```python
from build123d import *

# Parameters (mm, degrees)
SKETCH1_R           = 105
SKETCH1_R_2         = 20.325
BOSS_EXTRUDE1_DEPTH = 10
SKETCH2_R           = 6
CUT_EXTRUDE1_DEPTH  = 10
CIRPATTERN1_COUNT   = 6
SKETCH4_R           = 6
CUT_EXTRUDE2_DEPTH  = 10


with BuildPart() as part:
    # Sketch1 → Boss-Extrude1 (new body)
    with BuildSketch(Plane(origin=(0, 0, 0), x_dir=(1, 0, 0), z_dir=(0, 1, 0))):
        with Locations(Location((0, 0, 0), (0, 0, 270))):
            Circle(SKETCH1_R)
        with Locations(Location((0, 0, 0), (0, 0, 270))):
            Circle(SKETCH1_R_2, mode=Mode.SUBTRACT)
    extrude(amount=BOSS_EXTRUDE1_DEPTH)

    # Sketch2 → Cut-Extrude1 (cut)
    with BuildSketch(Plane(origin=(0, 10, 0), x_dir=(1, 0, 0), z_dir=(0, 1, 0))):
        with Locations(Location((93.00155101, 0.192929613, 0), (0, 0, 270))):
            Circle(SKETCH2_R)
        with Locations(Location((-46.333693559, -80.638170573, 0), (0, 0, 270))):
            Circle(SKETCH2_R)
        with Locations(Location((-46.667857451, 80.445240959, 0), (0, 0, 270))):
            Circle(SKETCH2_R)
    cut_extrude1 = extrude(amount=-CUT_EXTRUDE1_DEPTH, mode=Mode.SUBTRACT)

    # CirPattern1: Cut-Extrude1 ×6 about axis
    cirpattern1_axis = Axis((0, 0, 0), (0, 1, 0))
    for i in range(1, CIRPATTERN1_COUNT):
        add(cut_extrude1.rotate(cirpattern1_axis, i * 360 / CIRPATTERN1_COUNT), mode=Mode.SUBTRACT)

    # Sketch4 → Cut-Extrude2 (cut)
    with BuildSketch(Plane(origin=(0, 10, 0), x_dir=(1, 0, 0), z_dir=(0, 1, 0))):
        with Locations(Location((0, 80, 0), (0, 0, 270))):
            Circle(SKETCH4_R)
    extrude(amount=-CUT_EXTRUDE2_DEPTH, mode=Mode.SUBTRACT)


solid = part.part
```
The model under review builds one solid part; all positions refer to its coordinate system, in mm. Round coordinates to 2 decimals unless told otherwise and drop trailing zeros. Loops run counter-clockwise (first coordinate to the right, second up) from the corner with the lowest first, then second, coordinate; pieces in that order, holes last. Notation, with made-up numbers: (54, -14.75) -> (104, -14.75) arc R17 cw to (104, 14.25) -> close; hole circle Ø7 at (-5.75, 39.5). An arc over 180 degrees is marked (long way). Answer in a Markdown table with one row per item.
1) Consider section D-D, the plane y = 6.75. Count the separate pieces of the cut face and the enclosed holes in it, plus the area to 3 significant figures.
Taken from the geometry:
| item | result |
|---|---|
| separate pieces | 1 |
| enclosed holes | 8 |
| area | 32,500 mm² |
2) Consider section C-C, the plane x = 89.5. Write out the cut boundary in (y, z), plus the area to 3 significant figures.
Taken from the geometry:
| item | result |
|---|---|
| outline | (0, -54.91) -> (10, -54.91) -> (10, -5.07) -> (0, -5.07) -> close; (0, 4.68) -> (10, 4.68) -> (10, 54.91) -> (0, 54.91) -> close |
| area | 1,000 mm² |
3) For pin 1 Ø1.5 at (x, y) = (13, 1.5) entering from -Z; pin 2 Ø1.5 at (y, z) = (3, 64) entering from -X; pin 3 Ø1.5 at (y, z) = (5, 44.5) entering from +X, all flat-tipped, find the tip position at first contact; note any pin that passes through.
Taken from the geometry:
| item | result |
|---|---|
| pin 1 | stops at z = -104.28 |
| pin 2 | stops at x = -83.81 |
| pin 3 | stops at x = 95.45 |
4) Wall thickness on line 1 along X through (y, z) = (4.5, 0) (3 decimals); line 2 along Z through (x, y) = (1, 7); line 3 along X through (y, z) = (1.5, 78): over which ranges is each line inside the solid? List them lowest first.
Taken from the geometry:
| item | result |
|---|---|
| line 1 | x = -105 to -98.998, -87.005 to -20.325, 20.325 to 87.005, 98.998 to 105 |
| line 2 | z = -105 to -85.92, -74.08 to -20.3, 20.3 to 105 |
| line 3 | x = -70.29 to -51.72, -40.94 to 41.19, 52.15 to 70.29 |
5) Consider section B-B, the plane z = 0. Write out the cut boundary in (x, y) (3 decimals), plus the area to 3 significant figures.
Taken from the geometry:
| item | result |
|---|---|
| outline | (-105, 0) -> (-98.998, 0) -> (-98.998, 10) -> (-105, 10) -> close; (-87.005, 0) -> (-20.325, 0) -> (-20.325, 10) -> (-87.005, 10) -> close; (20.325, 0) -> (87.005, 0) -> (87.005, 10) -> (20.325, 10) -> close; (98.998, 0) -> (105, 0) -> (105, 10) -> (98.998, 10) -> close |
| area | 1,450 mm² |
6) Consider section A-A, the plane x = 0. Write out the cut boundary in (y, z) (3 decimals), plus the area to 3 significant figures.
Taken from the geometry:
| item | result |
|---|---|
| outline | (0, -105) -> (10, -105) -> (10, -86) -> (0, -86) -> close; (0, -74) -> (10, -74) -> (10, -20.325) -> (0, -20.325) -> close; (0, 20.325) -> (10, 20.325) -> (10, 105) -> (0, 105) -> close |
| area | 1,570 mm² |
7) Draft analysis for pull direction X (two halves, no side actions). For faces 1 (the flat face through (-22, 10, -1)), 2 (the cylindrical face through (31.54, 4.93, 100.15)), 3 (the cylindrical face through (-49.985, 5.07, 75.877)), state which applies: pulls with the +X half, pulls with the -X half, needs draft (parallel to the pull), parting line crosses it, or undercut.
Taken from the geometry:
| item | result |
|---|---|
| face 1 | needs draft |
| face 2 | parting line crosses it |
| face 3 | undercut |
